Could you check a few things on this model? Use its own coordinates, in mm. Face numbers are marked on the shaded views. A direction names the side the tool comes from. Give positions to 0.01 mm unless a question says otherwise; leave off trailing zeros. Loops run counter-clockwise (first coordinate to the right, second up) from the corner with the lowest first, then second, coordinate; pieces in that order, holes last. Notation, with made-up numbers: M 18.25,85.25 L 46.25,85.25 A22 cw 46.25,120.25 Z; hole C -10,-3 d8. An arc over 180 degrees is marked long. Use a Markdown table: item, result. Add a question column.
1) Suppose I cut it at C-C on y = -12.25. List the corners of the cut face in (x, z) for me, and give its area (3 significant figures).
2) Suppose I cut it at A-A on z = 12.5. List the corners of the cut face in (x, y) for me, and give its area (3 significant figures).
3) Suppose I cut it at D-D on z = 19.75. List the corners of the cut face in (x, y) for me, and give its area (3 significant figures).
4) Which directions (+Z, -Z, +X, -X, +Y, -Y) give clear straight access to the entire face, cutting with the end or side of a thin tool? Please do the marked faces 1, 2 and 3.
5) Will these pins go through, and if not, where does the flat tip stop? pin 1 Ø10 at (x, y) = (47, -3.5) entering from -Z; pin 2 Ø3 at (x, z) = (49, 14.5) entering from +Y; pin 3 Ø4.5 at (y, z) = (-7.5, 15.5) entering from -X; pin 4 Ø7.5 at (y, z) = (1, 11) entering from +X.
6) If I drill on line 1 along X through (y, z) = (-12.25, 12.5); line 2 along X through (y, z) = (4.5, 12.5); line 3 along Y through (x, z) = (50, 19.75), over which ranges is the centre line in solid material (lowest first)? Write a range as [from, to].
7) We'd pull the mould along Z, two halves only. Please class the marked faces 4, 5 and 6: +Z half, -Z half, draft (parallel to the pull), parting line (faces both ways), or undercut.
8) Suppose I cut it at B-B on x = 12.5. List the corners of the cut face in (y, z) for me.
```python
from build123d import *

# Parameters (mm, degrees)
BOSS_EXTRUDE1_DEPTH = 25
SKETCH3_R           = 11
CUT_EXTRUDE1_DEPTH  = 69.425214496
SKETCH4_R           = 4
CUT_EXTRUDE2_DEPTH  = 67.294871437


with BuildPart() as part:
    # Sketch2 → Boss-Extrude1 (new body)
    with BuildSketch(Plane.XY):
        with BuildLine():
            Line((0, 0), (0, 7))
            Line((0, 7), (31.5, 7))
            ThreePointArc((31.5, 7), (32.207106781, 6.707106781), (32.5, 6))
            Line((32.5, 6), (32.5, -9))
            ThreePointArc((32.5, -9), (32.792893219, -9.707106781), (33.5, -10))
            Line((33.5, -10), (59.000084567, -10))
            Line((59.000084567, -10), (59.000084567, -17))
            Line((59.000084567, -17), (27.520084567, -17))
            ThreePointArc((27.520084567, -17), (26.812977785, -16.707106781), (26.520084567, -16))
            Line((26.520084567, -16), (26.520084567, -1))
            ThreePointArc((26.520084567, -1), (26.227191348, -0.292893219), (25.520084567, 0))
            Line((25.520084567, 0), (0, 0))
        make_face()
    extrude(amount=BOSS_EXTRUDE1_DEPTH)

    # Sketch3 → Cut-Extrude1 (cut, through all)
    with BuildSketch(Plane(origin=(0, 7, 0), x_dir=(1, 0, 0), z_dir=(0, 1, 0))):
        with Locations(Location((12.5, -12.5, 0), (0, 0, 270))):
            Circle(SKETCH3_R)
    extrude(amount=-CUT_EXTRUDE1_DEPTH, mode=Mode.SUBTRACT)

    # Sketch4 → Cut-Extrude2 (cut, through all)
    with BuildSketch(Plane(origin=(0, -10, 0), x_dir=(1, 0, 0), z_dir=(0, 1, 0))):
        with Locations(Location((51.500084567, -12.5, 0), (0, 0, 270))):
            Circle(SKETCH4_R)
    extrude(amount=-CUT_EXTRUDE2_DEPTH, mode=Mode.SUBTRACT)


solid = part.part
```
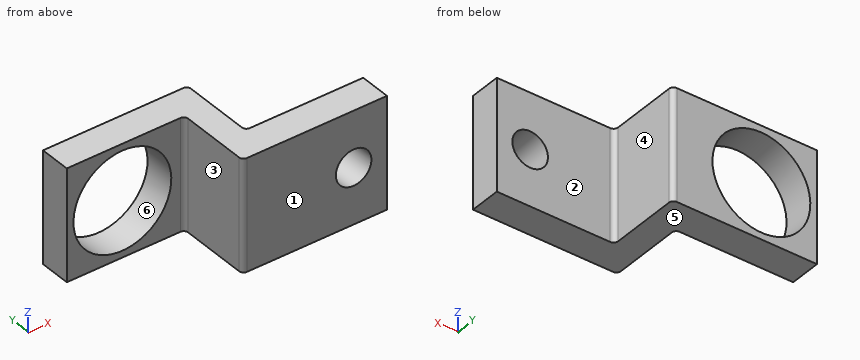
Answer block:
| question | item | result |
|---|---|---|
| 1 | outline | M 26.52,0 L 59,0 L 59,25 L 26.52,25 Z; hole C 51.5,12.5 d8 |
| 1 | area | 762 mm^2 |
| 2 | outline | M 0,0 L 1.5,0 L 1.5,7 L 0,7 Z; M 23.5,0 L 25.52,0 A1 cw 26.52,-1 L 26.52,-16 A1 ccw 27.52,-17 L 47.5,-17 L 47.5,-10 L 33.5,-10 A1 cw 32.5,-9 L 32.5,6 A1 ccw 31.5,7 L 23.5,7 Z; M 55.5,-17 L 59,-17 L 59,-10 L 55.5,-10 Z |
| 2 | area | 305 mm^2 |
| 3 | outline | M 0,0 L 4.23,0 L 4.23,7 L 0,7 Z; M 20.77,0 L 25.52,0 A1 cw 26.52,-1 L 26.52,-16 A1 ccw 27.52,-17 L 59,-17 L 59,-10 L 33.5,-10 A1 cw 32.5,-9 L 32.5,6 A1 ccw 31.5,7 L 20.77,7 Z |
| 3 | area | 399 mm^2 |
| 4 | face 1 | +Z, -Z, +X, -X, -Y |
| 4 | face 2 | +Z, -Z, +X, +Y |
| 4 | face 3 | +Z, -Z, -X, -Y |
| 5 | pin 1 | passes through |
| 5 | pin 2 | stops at y = -10 |
| 5 | pin 3 | stops at x = 26.52 |
| 5 | pin 4 | stops at x = 32.5 |
| 6 | line 1 | x = [26.52, 47.5], [55.5, 59] |
| 6 | line 2 | x = [0, 1.5], [23.5, 32.5] |
| 6 | line 3 | y = [-17, -10] |
| 7 | face 4 | draft |
| 7 | face 5 | -Z half |
| 7 | face 6 | undercut |
| 8 | outline | M 0,0 L 7,0 L 7,1.5 L 0,1.5 Z; M 0,23.5 L 7,23.5 L 7,25 L 0,25 Z |
